from build123d import *

# Parameters (mm, degrees)
SKETCH1_W           = 25.4
SKETCH1_H           = 38.1
SKETCH1_R           = 2.286
BOSS_EXTRUDE1_DEPTH = 3.81
BOSS_EXTRUDE2_DEPTH = 8.89
SKETCH3_W           = 13.97
SKETCH3_H           = 38.1
BOSS_EXTRUDE3_DEPTH = 2.54
CHAMFER1_SIZE       = 1.27
FILLET2_R           = 2.54


with BuildPart() as part:
    # Sketch1 → Boss-Extrude1 (new body)
    with BuildSketch(Plane(origin=(0, 0, 0), x_dir=(1, 0, 0), z_dir=(0, 1, 0))):
        with Locations((-7.112, -12.566479761)):
            Rectangle(SKETCH1_W, SKETCH1_H)
        with Locations(Location((-1.397, 1.276520239, 0), (0, 0, 90))):
            Circle(SKETCH1_R, mode=Mode.SUBTRACT)
        with Locations(Location((1.778, -27.298479761, 0), (0, 0, 90))):
            Circle(SKETCH1_R, mode=Mode.SUBTRACT)
    extrude(amount=BOSS_EXTRUDE1_DEPTH)

    # Sketch2 → Boss-Extrude2 (add)
    with BuildSketch(Plane(origin=(0, 3.81, 0), x_dir=(1, 0, 0), z_dir=(0, 1, 0))):
        Polygon((-19.812, 6.483520239), (-19.812, -31.616479761), (-5.842, -31.616479761), (-5.842, 6.483520239), (-8.382, 6.483520239), (-8.382, -29.076479761), (-17.272, -29.076479761), (-17.272, 6.483520239), align=None)
    extrude(amount=BOSS_EXTRUDE2_DEPTH)

    # Sketch3 → Boss-Extrude3 (add)
    with BuildSketch(Plane(origin=(0, 12.7, 0), x_dir=(1, 0, 0), z_dir=(0, 1, 0))):
        with Locations((-12.827, -12.566479761)):
            Rectangle(SKETCH3_W, SKETCH3_H)
    extrude(amount=BOSS_EXTRUDE3_DEPTH)

    # Chamfer1
    chamfer1_edges = [part.edges().sort_by_distance(p)[0] for p in [
        (-8.382, 12.7, 11.296479761),
        (-17.272, 12.7, 11.296479761),
    ]]
    chamfer(chamfer1_edges, length=CHAMFER1_SIZE)

    # Fillet2
    fillet2_edges = [part.edges().sort_by_distance(p)[0] for p in [
        (-19.812, 15.24, 12.566479761),
        (-5.842, 15.24, 12.566479761),
    ]]
    fillet(fillet2_edges, radius=FILLET2_R)


solid = part.part
For this review, take the finished solid that the model builds, in its own axes (mm). A direction names the side the tool comes from. Give positions to 0.01 mm unless a question says otherwise; leave off trailing zeros. Order: outer loops, then holes, each group sorted by start corner. A loop starts at its lowest first (then second) coordinate and runs counter-clockwise, first axis right, second up. Notation, with made-up numbers: (-35, -3) - (-20, -3) arc R7 ccw to (-20, 7) - close; hole circle Ø8 at (56, 72.5). An arc over 180 degrees is marked (long way). Answer as a JSON object with one key per item and string values. Group by question number.
Item 1: Take a section at B-B on x = -11.5. Give the boundary of the cut face in (y, z), and give its area (3 significant figures).
Item 2: Take a section at D-D on z = 24.5. Give the boundary of the cut face in (x, y), and give its area (3 significant figures).
Item 3: Wall thickness on line 1 along X through (y, z) = (10, 20.5); line 2 along Y through (x, z) = (-14.5, 18.5); line 3 along Y through (x, z) = (-4.25, 2.5): over which ranges is each line inside the solid? List them lowest first.
Item 4: Clearance check with flat-ended pins moving along their axes: pin 1 Ø4.5 at (y, z) = (9, 10) entering from +X; pin 2 Ø12.5 at (x, z) = (2, 9.5) entering from +Y; pin 3 Ø5 at (x, y) = (1, 7) entering from +Z; pin 4 Ø5 at (x, z) = (-12, 10) entering from -Y. State where each tip first meets the part, or that it passes through.
Item 5: Draft analysis for pull direction Y (two halves, no side actions). For faces 4 (the flat face through (0, 3.81, 12)), 5 (the flat face through (-13, 12.7, 11)), 6 (the cylindrical face through (-2.94, 1.88, 0.41)), state which applies: pulls with the +Y half, pulls with the -Y half, needs draft (parallel to the pull), parting line crosses it, or undercut.
Item 6: Take a section at A-A on z = 28.5. Give the boundary of the cut face in (x, y), and give its area (3 significant figures).
Item 7: Machinability: for faces 1 (the flat face through (-5.842, 8, 13)), 2 (the flat face through (-13, 3.81, 11)), 3 (the flat face through (-19.812, 6, 13)), which of the approach directions +Z, -Z, +X, -X, +Y, -Y give a long, thin tool a straight path to every point of the face, cutting with its end or side? Answer none if there is none.
Item 8: Take a section at C-C on y = 7.25. Give the boundary of the cut face in (x, z), and give its area (3 significant figures).
Reported:
{
 "1": {"outline": "(0, -6.48) - (3.81, -6.48) - (3.81, 29.08) - (12.7, 29.08) - (12.7, -6.48) - (15.24, -6.48) - (15.24, 31.62) - (0, 31.62) - close", "area": "265 mm^2"},
 "2": {"outline": "(-19.81, 0) - (5.59, 0) - (5.59, 3.81) - (-5.84, 3.81) - (-5.84, 12.7) arc R2.54 ccw to (-8.38, 15.24) - (-17.27, 15.24) arc R2.54 ccw to (-19.81, 12.7) - close; hole (-17.27, 3.81) - (-8.38, 3.81) - (-8.38, 11.43) - (-9.65, 12.7) - (-16, 12.7) - (-17.27, 11.43) - close", "area": "176 mm^2"},
 "3": {"line 1": "-19.81 to -17.27, -8.38 to -5.84", "line 2": "0 to 3.81, 12.7 to 15.24", "line 3": "0 to 3.81"},
 "4": {"pin 1": "x = -5.84", "pin 2": "y = 3.81", "pin 3": "through", "pin 4": "y = 0"},
 "5": {"face 4": "pulls with the +Y half", "face 5": "undercut", "face 6": "needs draft"},
 "6": {"outline": "(-19.81, 0) - (-0.17, 0) - (-0.17, 3.81) - (-5.84, 3.81) - (-5.84, 12.7) arc R2.54 ccw to (-8.38, 15.24) - (-17.27, 15.24) arc R2.54 ccw to (-19.81, 12.7) - close; (3.72, 0) - (5.59, 0) - (5.59, 3.81) - (3.72, 3.81) - close; hole (-17.27, 3.81) - (-8.38, 3.81) - (-8.38, 11.43) - (-9.65, 12.7) - (-16, 12.7) - (-17.27, 11.43) - close", "area": "161 mm^2"},
 "7": {"face 1": "+Z, -Z, +X, +Y", "face 2": "-Z", "face 3": "+Z, -Z, -X, +Y, -Y"},
 "8": {"outline": "(-19.81, -6.48) - (-17.27, -6.48) - (-17.27, 29.08) - (-8.38, 29.08) - (-8.38, -6.48) - (-5.84, -6.48) - (-5.84, 31.62) - (-19.81, 31.62) - close", "area": "216 mm^2"}
}
